```python
from build123d import *

# Parameters (mm, degrees)
PAD_DEPTH       = 58
SKETCH001_R     = 9.5
SKETCH001_R_2   = 7.6
PAD001_DEPTH    = 58
SKETCH002_R     = 7.6
SKETCH002_R_2   = 3
POCKET_DEPTH    = 58
SKETCH003_R     = 4.1
SKETCH003_W     = 9
SKETCH003_H     = 33
POCKET001_DEPTH = 53
SKETCH004_W     = 16
SKETCH004_H     = 16
POCKET002_DEPTH = 45
SKETCH005_W     = 16
SKETCH005_H     = 33
POCKET003_DEPTH = 40
SKETCH006_R     = 2.1
SKETCH006_R_2   = 1.6
POCKET004_DEPTH = 30
SKETCH007_R     = 3
SKETCH007_R_2   = 2.1
PAD002_DEPTH    = 5
SKETCH008_R     = 3
SKETCH008_R_2   = 2.1
PAD003_DEPTH    = 5
POCKET005_DEPTH = 58


with BuildPart() as part:
    # Sketch → Pad (new body)
    with BuildSketch(Plane.XY):
        Polygon((-33.20822, 18.829675), (19.79178, 18.829675), (19.79178, 2.829675), (3.79178, 2.829675), (-3.20822, -10.170325), (-11.20822, -10.170325), (-15.20822, -3.170325), (-15.20822, 2.829675), (-33.20822, 2.829675), align=None)
    extrude(amount=PAD_DEPTH)

    # Sketch001 → Pad001 (new body)
    with BuildSketch(Plane.XY.offset(58)):
        with Locations((10.29178, -3.670325)):
            Circle(SKETCH001_R)
        with Locations((10.29178, -3.670325)):
            Circle(SKETCH001_R_2, mode=Mode.SUBTRACT)
    extrude(amount=-PAD001_DEPTH)

    # Sketch002 → Pocket (cut)
    with BuildSketch(Plane.XY.offset(58)):
        with Locations((10.29178, -3.670325)):
            Circle(SKETCH002_R)
        with Locations((-6.70822, -3.670325)):
            Circle(SKETCH002_R_2)
    extrude(amount=-POCKET_DEPTH, mode=Mode.SUBTRACT)

    # Sketch003 → Pocket001 (cut)
    with BuildSketch(Plane.YZ.offset(19.79178)):
        with Locations((10.329675, 52.018545)):
            Circle(SKETCH003_R)
        with Locations((10.329675, 7.018545)):
            Circle(SKETCH003_R)
        with Locations((10.329675, 29.5)):
            Rectangle(SKETCH003_W, SKETCH003_H)
    extrude(amount=-POCKET001_DEPTH, mode=Mode.SUBTRACT)

    # Sketch004 → Pocket002 (cut)
    with BuildSketch(Plane.XY.offset(58)):
        with Locations((-7.20822, -5.170325)):
            Rectangle(SKETCH004_W, SKETCH004_H)
    extrude(amount=-POCKET002_DEPTH, mode=Mode.SUBTRACT)

    # Sketch005 → Pocket003 (cut)
    with BuildSketch(Plane.XZ.offset(-2.829675)):
        with Locations((-7.20822, 29.5)):
            Rectangle(SKETCH005_W, SKETCH005_H)
    extrude(amount=-POCKET003_DEPTH, mode=Mode.SUBTRACT)

    # Sketch006 → Pocket004 (cut)
    with BuildSketch(Plane.XZ.offset(-2.829675)):
        with Locations((-19.70822, 30)):
            Circle(SKETCH006_R)
        with Locations((-29.70822, 42)):
            Circle(SKETCH006_R_2)
        with Locations((-19.70822, 42)):
            Circle(SKETCH006_R_2)
    extrude(amount=-POCKET004_DEPTH, mode=Mode.SUBTRACT)

    # Sketch007 → Pad002 (new body)
    with BuildSketch(Plane.XZ.offset(-2.829675)):
        with Locations((-19.70822, 30)):
            Circle(SKETCH007_R)
        with Locations((-19.70822, 30)):
            Circle(SKETCH007_R_2, mode=Mode.SUBTRACT)
    extrude(amount=-PAD002_DEPTH)

    # Sketch008 → Pad003 (new body)
    with BuildSketch(Plane(origin=(0, 18.829675, 0), x_dir=(-1, 0, 0), z_dir=(0, 1, 0))):
        with Locations((19.70822, 30)):
            Circle(SKETCH008_R)
        with Locations((19.70822, 30)):
            Circle(SKETCH008_R_2, mode=Mode.SUBTRACT)
    extrude(amount=-PAD003_DEPTH)

    # Sketch009 → Pocket005 (cut)
    with BuildSketch(Plane.XY.offset(58)):
        Polygon((10.557791, -2.306743), (-0.062185, -9.183362), (0.481338, -10.022756), (11.101313, -3.146138), align=None)
    extrude(amount=-POCKET005_DEPTH, mode=Mode.SUBTRACT)


solid = part.part
```
Source: CAD feature listing. Evaluate the final solid. Frame: model axes, mm. A direction names the side the tool comes from. Give positions to 0.01 mm unless a question says otherwise; leave off trailing zeros. Loops run counter-clockwise (first coordinate to the right, second up) from the corner with the lowest first, then second, coordinate; pieces in that order, holes last. Notation, with made-up numbers: M 43.5,61 L 82.5,61 A20 ccw 82.5,87 Z; hole C 88.5,20 d3. An arc over 180 degrees is marked long. Put each result on its own line as item: value.
Q1. Mould query, pull axis X, two halves, no side actions, for faces 5 (the cylindrical face through (-5.32, -6.33, 6.59)), 6 (the flat face through (-15.208, 0, 6)), 7 (the flat face through (-7, -10.17, 6)). Classes: released by +X, released by -X, zero draft, split by the parting line, or undercut.
Response values:
face 5: undercut
face 6: released by -X
face 7: zero draft
Q2. Pin query (flat end, axial travel): P1, Ø4, axis at x = -19.71, z = 42, coming from the -Y side; P2, Ø10, axis at y = -5, z = 30.5, coming from the -X side; P3, Ø4, axis at y = -0.5, z = 42.5, coming from the +X side. Return the tip coordinate at first contact, or that it passes through.
Response values:
P1: stops at y = 2.83
P2: stops at x = 0.79
P3: stops at x = 19.72
Q3. Reachability of faces 1 (the flat face through (0.792, 1, 36)), 2 (the flat face through (-6, 11, 46)), 3 (the flat face through (3.104, -8.325, 29.406)), 4 (the flat face through (-20, 2.83, 36)) from +Z, -Z, +X, -X, +Y, -Y: full face, straight path, thin tool, end or side. Return the list, or none.
Response values:
face 1: -Y
face 2: none
face 3: +Z, -Z
face 4: +Z, -X, -Y
Q4. Section C-C (x = -20). Count the separate pieces of the cut face and the enclosed holes in it, and give its area (3 significant figures).
Response values:
separate pieces: 4
enclosed holes: 2
area: 480 mm²
Q5. Line query: probe 1 along X at (y, z) = (-3.5, 20.5); probe 2 along Y at (x, z) = (-5, 6); probe 3 along X at (y, z) = (-2, 9.5). Output: solid intervals per line, ascending. Write a range as [from, to].
Response values:
probe 1: x = [0.79, 2.69], [17.89, 19.79]
probe 2: y = [-10.17, -6.14], [-1.2, 6.36], [14.3, 18.83]
probe 3: x = [-15.21, -9.2], [-4.22, 2.88], [17.71, 19.64]
Q6. Section A-A (y = 7). Return the cut outline in (x, z).
Response values:
outline: M -33.21,0 L 19.79,0 L 19.79,4.63 L -33.21,4.63 Z; M -33.21,9.41 L 19.79,9.41 L 19.79,13 L -33.21,13 Z; M -33.21,46 L 19.79,46 L 19.79,49.63 L -33.21,49.63 Z; M -33.21,54.41 L 19.79,54.41 L 19.79,58 L -33.21,58 Z; C -19.71,30 d6; hole C -19.71,30 d4.2
Q7. Section B-B (z = 23.5). Return the cut outline in (x, y).
Response values:
outline: M -33.21,2.83 L -15.21,2.83 L -15.21,5.83 L -33.21,5.83 Z; M -33.21,14.83 L -15.21,14.83 L -15.21,18.83 L -33.21,18.83 Z; M 0.79,-2.74 L 0.85,-2.64 A9.5 ccw 1.82,-7.97 L 3.42,-6.93 A7.6 cw long 3.91,-7.8 L 2.32,-8.83 A9.5 ccw long 17.22,2.83 L 19.79,2.83 L 19.79,5.83 L 0.79,5.83 Z; M 0.79,14.83 L 19.79,14.83 L 19.79,18.83 L 0.79,18.83 Z
Q8. Section D-D (x = 7). Return the cut outline in (y, z), and give its area (3 significant figures).
Response values:
outline: M -12.58,0 L -10.52,0 L -10.52,58 L -12.58,58 Z; M 3.18,0 L 18.83,0 L 18.83,58 L 3.18,58 Z; hole M 5.83,13 L 14.83,13 L 14.83,46 L 5.83,46 Z; hole C 10.33,7.02 d8.2; hole C 10.33,52.02 d8.2
area: 625 mm²
